```python
from build123d import *

# Parameters (mm, degrees)
SALIENTE_EXTRUIR1_DEPTH = 26.3
REDONDEO1_R             = 1
REDONDEO2_R             = 2
REDONDEO3_R             = 13.1
CROQUIS2_R              = 5
CROQUIS2_R_2            = 1.675
CORTAR_EXTRUIR1_DEPTH   = 45.161663239
CROQUIS3_R              = 4
CROQUIS3_R_2            = 1.5
CORTAR_EXTRUIR2_DEPTH   = 50.313121927


with BuildPart() as part:
    # Croquis1 → Saliente-Extruir1 (new body)
    with BuildSketch(Plane(origin=(0, 0, 0), x_dir=(0, 0, -1), z_dir=(1, 0, 0))):
        Polygon((-17.25, 28.984375), (-14.25, 28.984375), (-14.25, -2.015625), (15.75, -2.015625), (15.75, -5.015625), (-17.25, -5.015625), align=None)
    extrude(amount=SALIENTE_EXTRUIR1_DEPTH)

    # Redondeo1
    redondeo1_edges = [part.edges().sort_by_distance(p)[0] for p in [
        (13.15, -2.015625, 14.25),
    ]]
    fillet(redondeo1_edges, radius=REDONDEO1_R)

    # Redondeo2
    redondeo2_edges = [part.edges().sort_by_distance(p)[0] for p in [
        (13.15, -5.015625, 17.25),
    ]]
    fillet(redondeo2_edges, radius=REDONDEO2_R)

    # Redondeo3
    redondeo3_edges = [part.edges().sort_by_distance(p)[0] for p in [
        (26.3, 28.984375, 15.75),
        (0, 28.984375, 15.75),
    ]]
    fillet(redondeo3_edges, radius=REDONDEO3_R)

    # Croquis2 → Cortar-Extruir1 (cut, through all)
    with BuildSketch(Plane(origin=(0, -2.015625, 0), x_dir=(1, 0, 0), z_dir=(0, 1, 0))):
        with Locations(Location((13, 1.75, 0), (0, 0, 270))):
            Circle(CROQUIS2_R)
        with Locations(Location((5.9, 8.3, 0), (0, 0, 270))):
            Circle(CROQUIS2_R_2)
        with Locations(Location((20.4, 8.3, 0), (0, 0, 270))):
            Circle(CROQUIS2_R_2)
        with Locations(Location((20.4, -4.8, 0), (0, 0, 270))):
            Circle(CROQUIS2_R_2)
        with Locations(Location((5.9, -4.8, 0), (0, 0, 270))):
            Circle(CROQUIS2_R_2)
    extrude(amount=-CORTAR_EXTRUIR1_DEPTH, mode=Mode.SUBTRACT)

    # Croquis3 → Cortar-Extruir2 (cut, through all)
    with BuildSketch(Plane(origin=(0, 0, 14.25), x_dir=(-1, 0, 0), z_dir=(0, 0, -1))):
        with Locations(Location((-13.2, 15.884375, 0), (0, 0, 90))):
            Circle(CROQUIS3_R)
        with Locations(Location((-21.7, 15.884375, 0), (0, 0, 90))):
            Circle(CROQUIS3_R_2)
        with Locations(Location((-4.7, 15.884375, 0), (0, 0, 90))):
            Circle(CROQUIS3_R_2)
    extrude(amount=-CORTAR_EXTRUIR2_DEPTH, mode=Mode.SUBTRACT)


solid = part.part
```
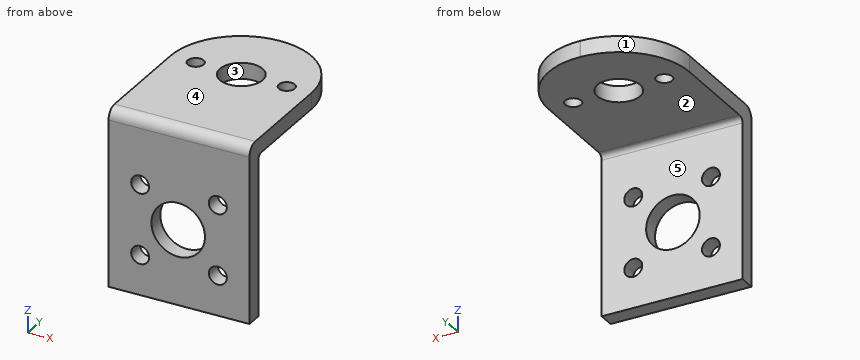
Here's how the part is built. I have some questions about the finished solid (model axes, mm). Face numbers are marked on the shaded views. A direction names the side the tool comes from. Round coordinates to 2 decimals unless told otherwise and drop trailing zeros. Order: outer loops, then holes, each group sorted by start corner. A loop starts at its lowest first (then second) coordinate and runs counter-clockwise, first axis right, second up. Notation, with made-up numbers: (-21.75, -20) -> (20.25, -20) arc R31 cw to (20.25, 6) -> close; hole circle Ø11 at (52, -33.5). An arc over 180 degrees is marked (long way). Use a Markdown table: item, result. Add a question column.
(1) Suppose I cut it at A-A, the plane z = -1.75. Please give me the cut outline in (x, y).
(2) If we mould it in two halves opening along Y, with no side actions, what happens to the marked faces 3, 4 and 5? For each: released by +Y, released by -Y, zero draft, split by the parting line, or undercut.
(3) Suppose I cut it at D-D, the plane x = 5.25. Please give me the cut outline in (y, z), and give its area (3 significant figures).
(4) Suppose I cut it at B-B, the plane z = -8.3. Please give me the cut outline in (x, y) (3 decimals), and give its area (3 significant figures).
(5) For pin 1 Ø10 at (x, z) = (14.5, 2.5) entering from -Y; pin 2 Ø3 at (x, y) = (6, 16.5) entering from -Z; pin 3 Ø5 at (x, z) = (5.5, 4) entering from +Y; pin 4 Ø7 at (x, y) = (13.2, 15.88) entering from -Z, each with a flat end and sliding along its axis, tell me the tip position at first contact or that it passes through.
(6) For the marked faces 1 and 2, which set-ups out of +Z, -Z, +X, -X, +Y, -Y let a thin tool reach every point of the face, with its end or its side?
(7) I need wall thicknesses on line 1 along X through (y, z) = (-3.5, 4.8) (3 decimals); line 2 along Y through (x, z) = (18.5, -11); line 3 along Z through (x, y) = (16.5, 10). Which ranges of each line are inside material? Lowest first, please.
(8) Suppose I cut it at C-C, the plane x = 10.25. Please give me the cut outline in (y, z).
Verdict:
| question | item | result |
|---|---|---|
| 1 | outline | (0, -5.02) -> (8, -5.02) -> (8, -2.02) -> (0, -2.02) -> close; (18, -5.02) -> (26.3, -5.02) -> (26.3, -2.02) -> (18, -2.02) -> close |
| 2 | face 3 | undercut |
| 2 | face 4 | zero draft |
| 2 | face 5 | released by +Y |
| 3 | outline | (-5.02, -15.75) -> (-2.02, -15.75) -> (-2.02, -9.84) -> (-5.02, -9.84) -> close; (-5.02, -6.76) -> (-2.02, -6.76) -> (-2.02, 3.26) -> (-5.02, 3.26) -> close; (-5.02, 6.34) -> (-2.02, 6.34) -> (-2.02, 13.25) arc R1 cw to (-1.02, 14.25) -> (14.49, 14.25) -> (14.49, 17.25) -> (-3.02, 17.25) arc R2 ccw to (-5.02, 15.25) -> close; (17.28, 14.25) -> (26.37, 14.25) -> (26.37, 17.25) -> (17.28, 17.25) -> close |
| 3 | area | 157 mm2 |
| 4 | outline | (0, -5.016) -> (4.225, -5.016) -> (4.225, -2.016) -> (0, -2.016) -> close; (7.575, -5.016) -> (18.725, -5.016) -> (18.725, -2.016) -> (7.575, -2.016) -> close; (22.075, -5.016) -> (26.3, -5.016) -> (26.3, -2.016) -> (22.075, -2.016) -> close |
| 4 | area | 58.8 mm2 |
| 5 | pin 1 | y = -5.02 |
| 5 | pin 2 | z = 14.25 |
| 5 | pin 3 | y = -2.02 |
| 5 | pin 4 | through |
| 6 | face 1 | +Z, -Z, -X, +Y |
| 6 | face 2 | -Z, +X, -X, +Y |
| 7 | line 1 | 0 to 4.225, 7.575 to 18.725, 22.075 to 26.3 |
| 7 | line 2 | -5.02 to -2.02 |
| 7 | line 3 | 14.25 to 17.25 |
| 8 | outline | (-5.02, -15.75) -> (-2.02, -15.75) -> (-2.02, -5.93) -> (-5.02, -5.93) -> close; (-5.02, 2.43) -> (-2.02, 2.43) -> (-2.02, 13.25) arc R1 cw to (-1.02, 14.25) -> (13.18, 14.25) -> (13.18, 17.25) -> (-3.02, 17.25) arc R2 ccw to (-5.02, 15.25) -> close; (18.59, 14.25) -> (28.67, 14.25) -> (28.67, 17.25) -> (18.59, 17.25) -> close |
